Input: dimensioned drawing with shaded views. Units: mm. Origin: part minimum x, y, z. A direction names the side the tool comes from. Give positions to 0.01 mm unless a question says otherwise; leave off trailing zeros. Order: outer loops, then holes, each group sorted by start corner. A loop starts at its lowest first (then second) coordinate and runs counter-clockwise, first axis right, second up.
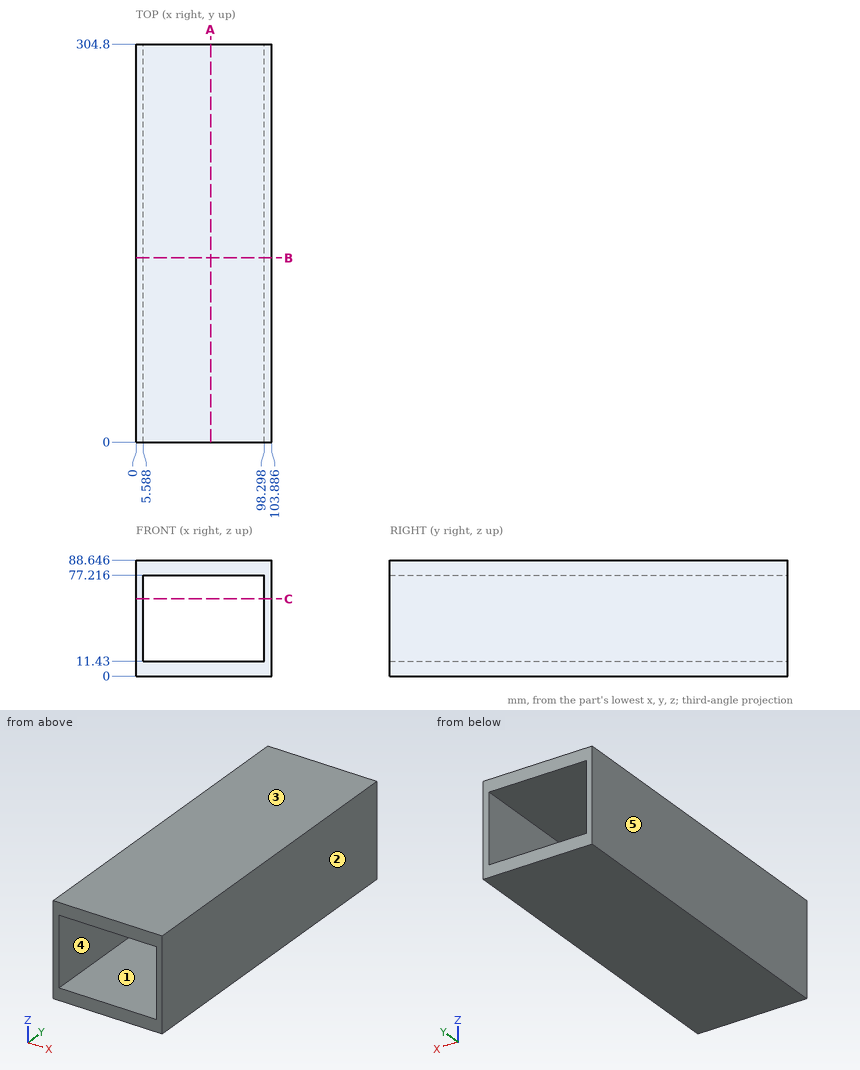
1) Material intervals for L1, parallel to X at y = 242.5, z = 57; L2, parallel to Z at x = 20.5, y = 80, sorted ascending.
Report:
L1: x = 0 to 5.59, 98.3 to 103.89
L2: z = 0 to 11.43, 77.22 to 88.65
2) Section query B-B, the plane y = 141. Return the cut outline in (x, z), and give its area (3 significant figures).
Report:
outline: (0, 0) - (103.89, 0) - (103.89, 88.65) - (0, 88.65) - close; hole (5.59, 11.43) - (98.3, 11.43) - (98.3, 77.22) - (5.59, 77.22) - close
area: 3,110 mm2
3) Section query A-A, the plane x = 57. Return the cut outline in (y, z).
Report:
outline: (0, 0) - (304.8, 0) - (304.8, 11.43) - (0, 11.43) - close; (0, 77.22) - (304.8, 77.22) - (304.8, 88.65) - (0, 88.65) - close
4) Section query C-C, the plane z = 59. Return the cut outline in (x, y), and give its area (3 significant figures).
Report:
outline: (0, 0) - (5.59, 0) - (5.59, 304.8) - (0, 304.8) - close; (98.3, 0) - (103.89, 0) - (103.89, 304.8) - (98.3, 304.8) - close
area: 3,410 mm2
5) Draft query along X for the marked faces 3, 4 and 5. Return one class per face: +X half, -X half, draft (parallel to the pull), parting line (faces both ways), or undercut.
Report:
face 3: draft
face 4: undercut
face 5: -X half
6) Reachability of the marked faces 1 and 2 from +Z, -Z, +X, -X, +Y, -Y: full face, straight path, thin tool, end or side. Return the list, or none.
Report:
face 1: +Y, -Y
face 2: +Z, -Z, +X, +Y, -Y
